Study the drawing (mm; zero at the part's minimum x, y, z) and answer. A direction names the side the tool comes from. Give positions to 0.01 mm unless a question says otherwise; leave off trailing zeros. Order: outer loops, then holes, each group sorted by start corner. A loop starts at its lowest first (then second) coordinate and runs counter-clockwise, first axis right, second up.
Item 1: Which of the six approach directions +Z, -Z, +X, -X, +Y, -Y give full straight-line access (tool end or side, diameter ignored) to the marked faces 1 and 2?
Item 2: A cutting plane is placed at B-B (x = 66). Write down the section's boundary in (y, z).
Item 3: A cutting plane is placed at D-D (x = 49). Write down the section's boundary in (y, z) (1 decimal).
Item 4: A cutting plane is placed at C-C (y = 112). Write down the section's boundary in (x, z) (1 decimal), plus the area to 3 significant figures.
Item 5: Find the intervals of material crossed by line 1 along X through (y, z) = (102, 16.5) (1 decimal); line 2 along Y through (x, z) = (42, 40.5); line 3 along Z through (x, y) = (43.5, 7) (1 decimal), in increasing order.
Item 6: A cutting plane is placed at A-A (z = 51). Write down the section's boundary in (x, y) (1 decimal).
Item 7: Given pin 1 Ø10 at (x, y) = (87.5, 72) entering from +Z, flat-ended and moving along its own axis, determine where the tip first touches the part or whether it passes through.
Item 8: The mould has two halves that part along Y. Classify the marked faces 3, 4, 5 and 6: +Y half, -Y half, draft (parallel to the pull), parting line (faces both ways), or undercut.
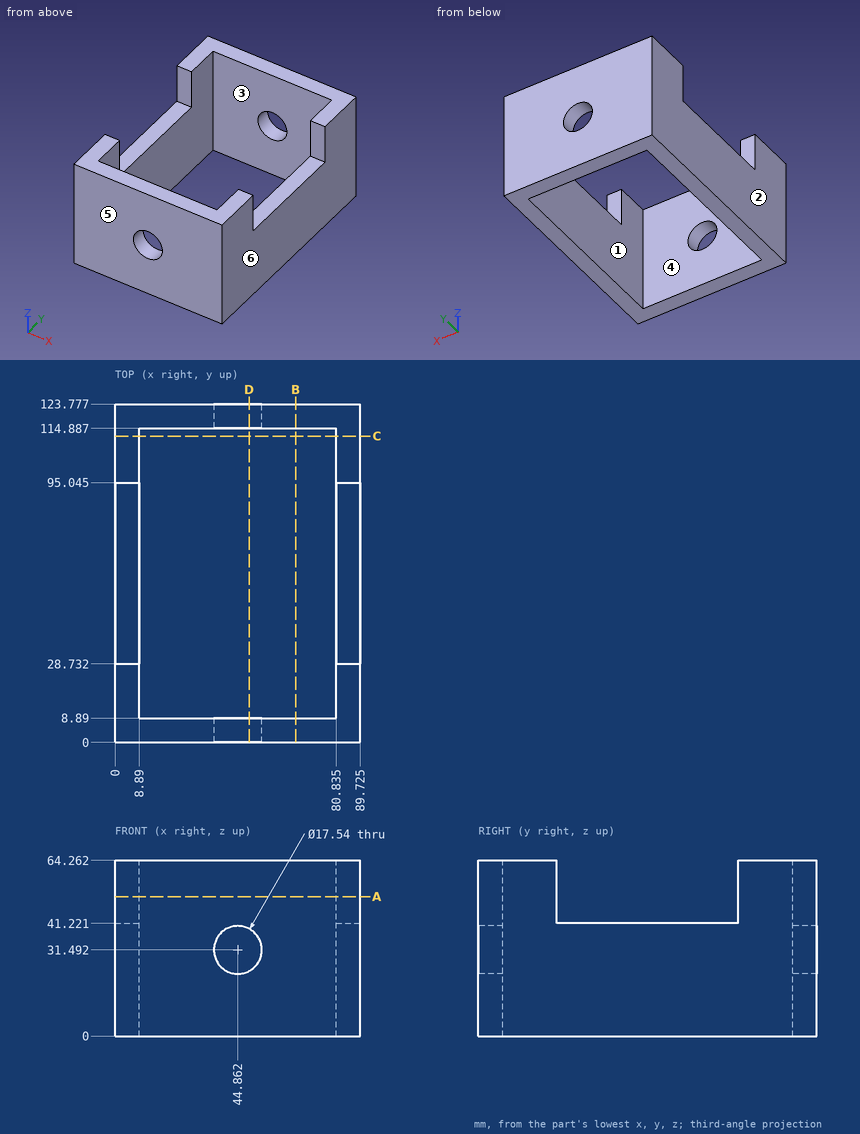
Response values:
1. face 1: +Z, -Z
1. face 2: +Z, -Z, -X, +Y, -Y
2. outline: (0, 0) - (8.89, 0) - (8.89, 64.26) - (0, 64.26) - close; (114.89, 0) - (123.78, 0) - (123.78, 64.26) - (114.89, 64.26) - close
3. outline: (0, 0) - (8.9, 0) - (8.9, 23.8) - (0, 23.8) - close; (0, 39.2) - (8.9, 39.2) - (8.9, 64.3) - (0, 64.3) - close; (114.9, 0) - (123.8, 0) - (123.8, 23.8) - (114.9, 23.8) - close; (114.9, 39.2) - (123.8, 39.2) - (123.8, 64.3) - (114.9, 64.3) - close
4. outline: (0, 0) - (8.9, 0) - (8.9, 64.3) - (0, 64.3) - close; (80.8, 0) - (89.7, 0) - (89.7, 64.3) - (80.8, 64.3) - close
4. area: 1,140 mm2
5. line 1: x = 0 to 8.9, 80.8 to 89.7
5. line 2: y = 0 to 8.89, 114.89 to 123.78
5. line 3: z = 0 to 22.8, 40.2 to 64.3
6. outline: (0, 0) - (89.7, 0) - (89.7, 28.7) - (80.8, 28.7) - (80.8, 8.9) - (8.9, 8.9) - (8.9, 28.7) - (0, 28.7) - close; (0, 95) - (8.9, 95) - (8.9, 114.9) - (80.8, 114.9) - (80.8, 95) - (89.7, 95) - (89.7, 123.8) - (0, 123.8) - close
7. pin 1: stops at z = 41.22
8. face 3: undercut
8. face 4: undercut
8. face 5: -Y half
8. face 6: draft
